Geometry: final body of the model. Coordinates: model frame, mm. A direction names the side the tool comes from. Give positions to 0.01 mm unless a question says otherwise; leave off trailing zeros. Write each loop counter-clockwise with the first axis right and the second up, starting at its lowest first coordinate (ties: lowest second). Pieces come first, ordered by that corner, then holes. Notation, with made-up numbers: M 37,22 L 79,22 A29 cw 79,45 Z; hole C 39.25,56.5 d10. An arc over 180 degrees is marked long. Use a Markdown table: item, result. Add a question column.
1) Section A-A on y = -17.5. Return the cut outline in (x, z).
2) Draft query along X for faces 3 (the cylindrical face through (11.93, -15.21, -5.9)), 4 (the conical face through (-4.566, -11.759, -0.019)), 5 (the cylindrical face through (-0.18, -0.86, 5.6)). Return one class per face: +X half, -X half, draft (parallel to the pull), parting line (faces both ways), or undercut.
3) Set-up query: faces 1 (the cylindrical face through (7.385, -21.122, -0.751)), 2 (the flat face through (0, -30, 0)). Return all of +Z, -Z, +X, -X, +Y, -Y with unobstructed straight access to the full face (end or side cutting, diameter ignored); none if empty.
4) Section B-B on y = -12.5. Return the cut outline in (x, z), then the cut area to 3 significant figures.
5) Line query: line 1 (X direction, y = -28, z = 1.25); line 2 (X direction, y = -24, z = -2.25); line 3 (Z direction, x = 5, y = -21.25). Output: solid intervals per line, ascending.
6) Pin query (flat end, axial travel): pin 1 (2 mm diameter, centred on x = 9.5, z = -2.5, fed in from +Y); pin 2 (1.5 mm diameter, centred on x = -4, y = -26, fed in from +Z). Return the tip coordinate at first contact, or that it passes through.
```python
from build123d import *

# Parameters (mm, degrees)
SKETCH1_W                   = 25
SKETCH1_H                   = 13
BOSS_EXTRUDE1_DEPTH         = 30
FILLET1_R                   = 2
FILLET2_R                   = 3
M6_TAPPED_HOLE1_D           = 5
M6_TAPPED_HOLE1_DEPTH       = 17
M6_TAPPED_HOLE1_CSINK_D     = 6.05
M6_TAPPED_HOLE1_CSINK_ANGLE = 90
M6_TAPPED_HOLE1_TIP         = 1.502151548
CUT_EXTRUDE1_DEPTH          = 7.5


with BuildPart() as part:
    # Sketch1 → Boss-Extrude1 (new body)
    with BuildSketch(Plane(origin=(0, 0, 0), x_dir=(1, 0, 0), z_dir=(0, 1, 0))):
        Rectangle(SKETCH1_W, SKETCH1_H)
    extrude(amount=-BOSS_EXTRUDE1_DEPTH)

    # Fillet1
    fillet1_edges = [part.edges().sort_by_distance(p)[0] for p in [
        (12.5, -15, 6.5),
        (-12.5, -15, 6.5),
        (-12.5, -15, -6.5),
        (12.5, -15, -6.5),
    ]]
    fillet(fillet1_edges, radius=FILLET1_R)

    # Fillet2
    # the kernel refuses this fillet: 3 mm, written as the material it takes off along each edge
    with BuildSketch(Plane(origin=(-18, 0, 6.5), x_dir=(0, -1, 0), z_dir=(1, 0, 0))) as fillet2_piece_1:
        with BuildLine():
            CenterArc((FILLET2_R, FILLET2_R), FILLET2_R, 180, 90)
            Line((0, FILLET2_R), (0, 0))
            Line((0, 0), (FILLET2_R, 0))
        make_face()
    extrude(amount=36, mode=Mode.SUBTRACT)

    # M6 Tapped Hole1
    with Locations(Plane(origin=(0, -30, 0), x_dir=(-1, 0, 0), z_dir=(0, -1, 0))):
        with Locations((-5, 0), (5, 0)):
            CounterSinkHole(M6_TAPPED_HOLE1_D / 2, M6_TAPPED_HOLE1_CSINK_D / 2, depth=M6_TAPPED_HOLE1_DEPTH, counter_sink_angle=M6_TAPPED_HOLE1_CSINK_ANGLE)
            with Locations((0, 0, -(M6_TAPPED_HOLE1_DEPTH + M6_TAPPED_HOLE1_TIP / 2))):  # 118° drill point
                Cone(0, M6_TAPPED_HOLE1_D / 2, M6_TAPPED_HOLE1_TIP, mode=Mode.SUBTRACT)

    # Sketch5 → Cut-Extrude1 (cut, symmetric)
    with BuildSketch(Plane(origin=(0, 0, 0), x_dir=(0, 0, -1), z_dir=(1, 0, 0))):
        Polygon((-6.5, -8), (-6.115988572, -30), (-6.5, -30), align=None)
    extrude(amount=CUT_EXTRUDE1_DEPTH, both=True, mode=Mode.SUBTRACT)


solid = part.part
```
Found:
| question | item | result |
|---|---|---|
| 1 | outline | M -12.5,-4.5 A2 ccw -10.5,-6.5 L 10.5,-6.5 A2 ccw 12.5,-4.5 L 12.5,4.5 A2 ccw 10.5,6.5 L 7.5,6.5 L 7.5,6.33 L -7.5,6.33 L -7.5,6.5 L -10.5,6.5 A2 ccw -12.5,4.5 Z; hole C -5,0 d5; hole C 5,0 d5 |
| 2 | face 3 | +X half |
| 2 | face 4 | undercut |
| 2 | face 5 | draft |
| 3 | face 1 | -Y |
| 3 | face 2 | +Z, -Z, +X, -X, -Y |
| 4 | outline | M -12.5,-4.5 A2 ccw -10.5,-6.5 L 10.5,-6.5 A2 ccw 12.5,-4.5 L 12.5,4.5 A2 ccw 10.5,6.5 L 7.5,6.5 L 7.5,6.42 L -7.5,6.42 L -7.5,6.5 L -10.5,6.5 A2 ccw -12.5,4.5 Z; hole C -5,0 d3.34; hole C 5,0 d3.34 |
| 4 | area | 303 mm² |
| 5 | line 1 | -12.5 to -7.17, -2.83 to 2.83, 7.17 to 12.5 |
| 5 | line 2 | -12.5 to -6.09, -3.91 to 3.91, 6.09 to 12.5 |
| 5 | line 3 | -6.5 to -2.5, 2.5 to 6.27 |
| 6 | pin 1 | y = 0 |
| 6 | pin 2 | z = 6.2 |
